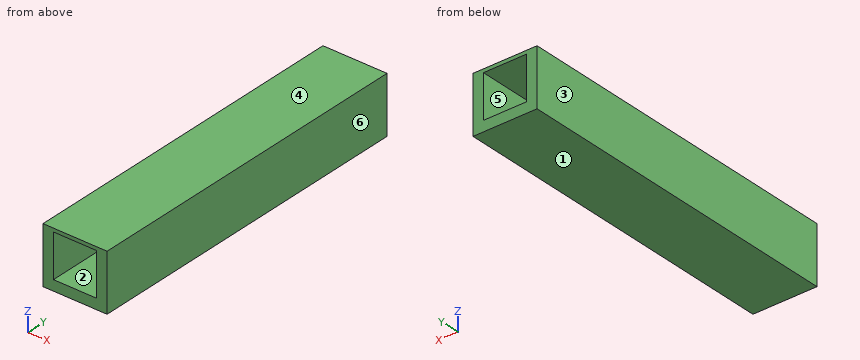
Autodesk Fusion 360 part; units mm, degrees
sketch "Sketch1" plane through (0, 0, 0) normal (0, 0, 1) x (1, 0, 0)
  line L0 (0, 0) -> (17, 0)
  line L1 (17, 0) -> (17, 200)
  line L2 (17, 200) -> (0, 200)
  line L3 (0, 200) -> (0, 0)
  line L4 (5, 0) -> (5, 200)
  line L5 (12, 0) -> (12, 200)
  dimension "d1" = 17
  dimension "d2" = 200
  dimension "d3" = 200
  dimension "d4" = 7
  dimension "d5" = 200
extrude "Extrude1" add sketch "Sketch1" along normal blind 5
sketch "Sketch2" plane through (0, 0, 5) normal (0, 0, 1) x (-1, 0, 0)
  line L0 (0, -200) -> (0, 0)
  line L1 (0, 0) -> (-17, 0)
  line L2 (-17, 0) -> (-17, -200)
  line L3 (-17, -200) -> (0, -200)
  line L4 (-5, 0) -> (-5, -200)
  line L5 (-12, 0) -> (-12, -200)
  dimension "d8" = 5
  dimension "d9" = 7
  dimension "d10" = 200
  dimension "d11" = 200
extrude "Extrude2" add sketch "Sketch2" along normal blind 12 contours L0 L1 L3 L4 | L1 L2 L3 L5
sketch "Sketch3" plane through (12, 0, 0) normal (-1, 0, 0) x (0, -1, 0)
  line L0 (-200, 5) -> (0, 5)
  line L1 (0, 5) -> (0, 17)
  line L2 (0, 17) -> (-200, 17)
  line L3 (-200, 17) -> (-200, 5)
  line L4 (0, 17) -> (0, 12)
  line L5 (0, 12) -> (-200, 12)
  dimension "d14" = 200
extrude "Extrude3" add sketch "Sketch3" along normal blind 7 contours L1 L2 L3 L4 L5
move_face "OffsetFaces1" offset -0.5 4 faces at (12, 133.3333, 9.6667) (9.6667, 66.6667, 12) (5, 133.3333, 9.6667) (7.3333, 133.3333, 5)
sketch "Sketch4" plane through (0, 0, 17) normal (0, 0, 1) x (-1, 0, 0)
  line L0 (-17, -200) -> (0, -200)
  line L1 (0, -200) -> (0, 0)
  line L2 (0, 0) -> (-17, 0)
  line L3 (-17, 0) -> (-17, -200)
  line L4 (25, 0) -> (25, -200)
  line L5 (-42, 0) -> (-42, -200)
  line L6 (25, -200) -> (-42, -200)
  line L7 (25, 0) -> (-42, 0)
  dimension "d18" = 25
  dimension "d19" = 25
extrude "Extrude4" add sketch "Sketch4" along normal blind 2.5
move_face "OffsetFaces2" offset -3 3 faces at (17, 133.3333, 11.3333) (5.6667, 133.3333, 0) (0, 133.3333, 5.6667)
move_face "MoveFace1" by (0, 0, 3) 4 faces at (9.8333, 66.6667, 12.5) (4.5, 133.3333, 9.8333) (7.1667, 133.3333, 4.5) (12.5, 133.3333, 9.8333)
extrude "Extrude5" cut 1 faces at (6.6667, 133.3333, 3) along direction (0, 0, 1) blind 3
extrude "Extrude6" cut 1 faces at (19.6667, 133.3333, 19.5) along direction (0, 0, -1) blind 1
move_face "OffsetFaces3" offset 0.5 4 faces at (12.5, 133.3333, 12.8333) (7.1667, 133.3333, 7.5) (9.8333, 66.6667, 15.5) (4.5, 133.3333, 12.8333)
move_face "OffsetFaces4" offset 1 4 faces at (5, 133.3333, 12.6667) (7.3333, 133.3333, 8) (12, 133.3333, 12.6667) (7.3333, 66.6667, 15)
move_face "OffsetFaces5" offset -0.5 4 faces at (11, 133.3333, 12.3333) (9.3333, 66.6667, 14) (6, 133.3333, 12.3333) (7.6667, 133.3333, 9)
move_face "OffsetFaces6" offset -0.5 3 faces at (14, 66.6667, 9.6667) (6.6667, 133.3333, 6) (3, 66.6667, 13.3333)
move_face "OffsetFaces7" offset -0.5 3 faces at (13.5, 66.6667, 10) (6.8333, 133.3333, 6.5) (3.5, 66.6667, 13.5)
move_face "OffsetFaces8" offset -0.5 3 faces at (13, 66.6667, 10.3333) (7, 133.3333, 7) (4, 66.6667, 13.6667)
move_face "MoveFace2" by (0, 0, 3) 4 faces at (11.5, 133.3333, 12.5) (7.5, 66.6667, 14.5) (7.5, 133.3333, 8.5) (5.5, 133.3333, 12.5)
move_face "OffsetFaces9" offset -3 1 faces at (7.1667, 133.3333, 7.5)
move_face "OffsetFaces10" offset -0.5 2 faces at (32.1667, 133.3333, 17) (-5.3333, 66.6667, 17)
extrude "Extrude7" add 1 faces at (7.1667, 133.3333, 10.5) along direction (0, 0, -1) blind 0.5
move_face "MoveFace3" by (0, 0, -0.5) 4 faces at (11.5, 66.6667, 13.5) (7.5, 66.6667, 17.5) (5.5, 66.6667, 13.5) (7.5, 133.3333, 11.5)
move_face "OffsetFaces11" offset -4.5 1 faces at (42, 66.6667, 17.8333)
move_face "OffsetFaces12" offset -4.5 1 faces at (-25, 66.6667, 17.8333)
move_face "OffsetFaces13" offset 50 1 faces at (7.1667, 0, 18.1667)
move_face "OffsetFaces14" offset -0.5 4 faces at (11.5, 116.6667, 15) (7.5, 116.6667, 11) (5.5, 116.6667, 15) (9.5, 33.3333, 17)
move_face "OffsetFaces15" offset 0.5 3 faces at (12.5, 33.3333, 12.5) (7.1667, 116.6667, 10) (4.5, 116.6667, 15)
move_face "OffsetFaces16" offset 0.5 1 faces at (10, 33.3333, 9.5)
move_face "MoveFace4" by (0, 0, -0.5) 4 faces at (12, 33.3333, 15.1667) (9.6667, 33.3333, 10.5) (5, 33.3333, 15.1667) (7.3333, 116.6667, 17.5)
move_face "OffsetFaces17" offset 0.5 4 faces at (12, 33.3333, 14.6667) (7.3333, 116.6667, 17) (5, 33.3333, 14.6667) (9.6667, 33.3333, 10)
move_face "MoveFace5" by (0, 0, 0.5) 4 faces at (5.5, 116.6667, 14.5) (7.5, 116.6667, 10.5) (11.5, 116.6667, 14.5) (9.5, 33.3333, 16.5)
move_face "OffsetFaces18" offset -0.5 1 faces at (10, 33.3333, 9)
move_face "OffsetFaces19" offset -0.02 1 faces at (7.5, 116.6667, 11)
move_face "OffsetFaces20" offset -0.2 2 faces at (11.5, 116.6667, 14.9933) (5.5, 116.6667, 14.9933)
move_face "OffsetFaces21" offset -0.18 2 faces at (9.5667, 33.3333, 17) (7.4333, 116.6667, 10.98)
move_face "OffsetFaces22" offset 0.18 1 faces at (9.5667, 33.3333, 17.18)
move_face "OffsetFaces23" offset 0.1 2 faces at (11.7, 33.3333, 12.8667) (5.3, 33.3333, 12.8667)
move_face "OffsetFaces24" offset 0.1 2 faces at (13, 116.6667, 14.8333) (4, 33.3333, 12.1667)
move_face "OffsetFaces25" offset 0.2 1 faces at (6.9667, 116.6667, 9.5)
move_face "OffsetFaces26" offset -1 1 faces at (18.1667, 116.6667, 18.5)
move_face "OffsetFaces27" offset -202.2 1 faces at (7.4667, -50, 9.8)
move_face "OffsetFaces28" offset 1 1 faces at (7.4667, 152.2, 9.8)
The listing builds one solid part. Answer for the finished solid, in the listing's coordinates (mm). Face numbers are marked on the shaded views. A direction names the side the tool comes from. Coordinates: 2 decimals unless noted, no trailing zeros. Write each loop counter-clockwise with the first axis right and the second up, starting at its lowest first coordinate (ties: lowest second). Pieces come first, ordered by that corner, then holes. Notation, with made-up numbers: (-2, 32.5) - (46, 32.5) arc R35 cw to (46, 69.5) - close; hole circle Ø8 at (0.5, 36). An arc over 180 degrees is marked (long way). One line per item, written item: value.
1) Consider line 1 along X through (y, z) = (192, 11.25); line 2 along Z through (x, y) = (11.5, 188). Determine where each line is inside the solid, lowest interval first. Write a range as from..to.
Geometry check:
line 1: x = 3.9..5.4, 11.6..13.1
line 2: z = 9.3..10.8, 17..17.5
2) Find section B-B (x = 10.25). Give the vertices of the cut face in (y, z).
Geometry check:
outline: (151.2, 9.3) - (200, 9.3) - (200, 10.8) - (151.2, 10.8) - close; (151.2, 17) - (200, 17) - (200, 17.5) - (151.2, 17.5) - close
3) For a pull along X with two mould halves and no side action, classify the marked faces 3, 4, 5 and 6 as pulls with the +X half, pulls with the -X half, needs draft (parallel to the pull), parting line crosses it, or undercut.
Geometry check:
face 3: pulls with the -X half
face 4: needs draft
face 5: undercut
face 6: pulls with the +X half
4) Find section C-C (y = 171.5). Give the vertices of the cut face in (x, z), and give its area (3 significant figures).
Geometry check:
outline: (3.9, 9.3) - (13.1, 9.3) - (13.1, 17.5) - (3.9, 17.5) - close; hole (5.4, 10.8) - (11.6, 10.8) - (11.6, 17) - (5.4, 17) - close
area: 37.0 mm2
5) Find section A-A (z = 12.5). Give the vertices of the cut face in (x, y).
Geometry check:
outline: (3.9, 151.2) - (5.4, 151.2) - (5.4, 200) - (3.9, 200) - close; (11.6, 151.2) - (13.1, 151.2) - (13.1, 200) - (11.6, 200) - close
6) A tool of negligible diameter and unlimited length cuts with its end or side. For the marked faces 1 and 2, from which of +Z, -Z, +X, -X, +Y, -Y can it reach the whole face along a straight path? Write none if from no direction.
Geometry check:
face 1: -Z, +X, -X, +Y, -Y
face 2: +Y, -Y
